from build123d import *

# Parameters (mm, degrees)
PAD_DEPTH       = 420
THICKNESS_T     = -5
SKETCH001_W     = 175
SKETCH001_H     = 410
POCKET_DEPTH    = 13
SKETCH002_W     = 96.930253
SKETCH002_H     = 26.478514
POCKET001_DEPTH = 8
SKETCH003_W     = 162
SKETCH003_H     = 2.108998
PAD001_DEPTH    = 180


with BuildPart() as part:
    # Sketch → Pad (new body)
    with BuildSketch(Plane.YZ):
        Polygon((-196.253947, 0), (-23.746053, 0), (0, 6.755281), (0, 55.271607), (-18.174265, 68.847916), (-201.591564, 44.70057), (-220, 31.443514), (-220, 6.755281), align=None)
    extrude(amount=PAD_DEPTH)

    # Thickness
    thickness_openings = [part.faces().sort_by_distance(p)[0] for p in [
        (210, -109.882914, 56.774243),
    ]]
    offset(amount=THICKNESS_T, openings=thickness_openings, kind=Kind.INTERSECTION)

    # Sketch001 (on Face5 of Pad) → Pocket (cut)
    with BuildSketch(Plane(origin=(0, -9.219212, 70.026871), x_dir=(0, -0.991445, -0.130526), z_dir=(0, -0.130526, 0.991445))):
        with Locations((101.532325, 210)):
            Rectangle(SKETCH001_W, SKETCH001_H)
    extrude(amount=-POCKET_DEPTH, mode=Mode.SUBTRACT)

    # Sketch002 (on Face5 of Pocket) → Pocket001 (cut)
    with BuildSketch(Plane.YZ.offset(420)):
        with Locations((-120.639269, 25.939101)):
            Rectangle(SKETCH002_W, SKETCH002_H)
    extrude(amount=-POCKET001_DEPTH, mode=Mode.SUBTRACT)

    # Sketch003 (on Face13 of Pocket001) → Pad001 (join)
    with BuildSketch(Plane(origin=(0, -13.912277, -1.831586), x_dir=(1, 0, 0), z_dir=(0, -0.991445, -0.130526))):
        with Locations((334, 69.576631)):
            Rectangle(SKETCH003_W, SKETCH003_H)
    extrude(amount=PAD001_DEPTH)


solid = part.part
For this review, take the finished solid that the model builds, in its own axes (mm). A direction names the side the tool comes from. Coordinates: 2 decimals unless noted, no trailing zeros. Order: outer loops, then holes, each group sorted by start corner. A loop starts at its lowest first (then second) coordinate and runs counter-clockwise, first axis right, second up. Notation, with made-up numbers: (6.25, 26.25) -> (59.25, 26.25) arc R31 cw to (59.25, 52.25) -> close; hole circle Ø5 at (-30, 39). An arc over 180 degrees is marked (long way). Return JSON: item names as keys, results as strings.
1. For line 1 (Y direction, x = 317, z = 26); line 2 (X direction, y = -31, z = 46); line 3 (Z direction, x = 213, y = -113.5), list the stretches that pass through material, from the lowest coordinate up. Write a range as from..to.
Answer block:
{"line 1": "-220..-215, -5..0", "line 2": "0..5, 415..420", "line 3": "0..5"}
2. Machinability: for faces 1 (the flat face through (420, -87, 43)), 2 (the flat face through (5, -109, 33)), which of the approach directions +Z, -Z, +X, -X, +Y, -Y give a long, thin tool a straight path to every point of the face, cutting with its end or side? Answer none if there is none.
Answer block:
{"face 1": "+Z, -Z, +X, +Y, -Y", "face 2": "none"}
3. We need section C-C on z = 20.5. Write out the cut boundary in (x, y), and give its area (3 significant figures).
Answer block:
{"outline": "(0, -220) -> (420, -220) -> (420, -169.1) -> (415, -169.1) -> (415, -215) -> (5, -215) -> (5, -5) -> (415, -5) -> (415, -72.17) -> (420, -72.17) -> (420, 0) -> (0, 0) -> close", "area": "5,820 mm²"}
4. We need section D-D on y = -13. Write out the cut boundary in (x, z), and give its area (3 significant figures).
Answer block:
{"outline": "(0, 3.06) -> (420, 3.06) -> (420, 64.98) -> (0, 64.98) -> close; hole (5, 8.26) -> (415, 8.26) -> (415, 58.74) -> (5, 58.74) -> close", "area": "5,310 mm²"}
5. The part is to be moulded in two halves that separate along X. For faces 3 (the flat face through (207.06, -208.293, 3.425)), 4 (the flat face through (207.13, -13.8, 59.34)), 5 (the flat face through (0, -112, 27)), 6 (the flat face through (207.13, -205.49, 35.73)), say which applies: +X half, -X half, draft (parallel to the pull), parting line (faces both ways), or undercut.
Answer block:
{"face 3": "draft", "face 4": "undercut", "face 5": "-X half", "face 6": "undercut"}
6. For pin 1 Ø1 at (x, y) = (51, -44.5) entering from +Z; pin 2 Ø1 at (x, y) = (346, -27) entering from +Z; pin 3 Ø1.5 at (x, y) = (418, -125.5) entering from +Z, all flat-tipped, find the tip position at first contact; note any pin that passes through.
Answer block:
{"pin 1": "z = 5", "pin 2": "z = 67.75", "pin 3": "z = 54.82"}
